```python
from build123d import *

# Parameters (mm, degrees)
F2_R     = 75
F3_DEPTH = 4
F5_R     = 67.5
F6_DEPTH = 12
F8_R     = 75
F9_DEPTH = 4


with BuildPart() as f3:
    # F2 (on Top) → F3 (new body)
    with BuildSketch(Plane.XY):
        Circle(F2_R)
    extrude(amount=F3_DEPTH)

    # F5 (on offset) → F6 (join)
    with BuildSketch(Plane.XY.offset(4)):
        Circle(F5_R)
    extrude(amount=F6_DEPTH)

    # F8 (on offset) → F9 (join)
    with BuildSketch(Plane.XY.offset(16)):
        Circle(F8_R)
    extrude(amount=F9_DEPTH)


with BuildPart() as f10_1:
    # F10: copy of F3
    add(f3.part.moved(Location((0, 0, 20))))


with BuildPart() as f12_1:
    # F12: copy of F3
    add(f3.part)


solid = f3.part
```
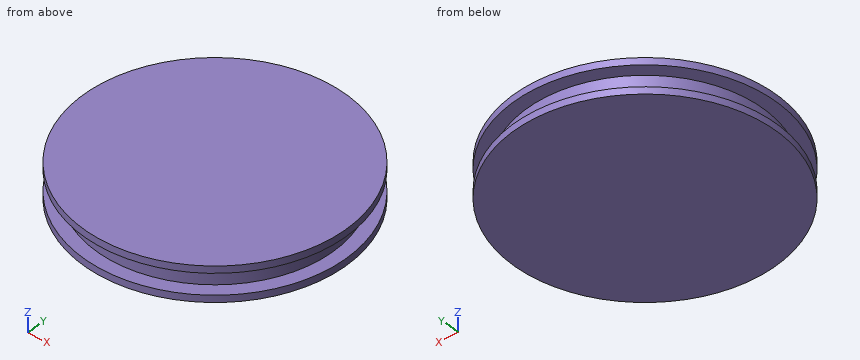
Could you check a few things on this model? Use its own coordinates, in mm. Coordinates: 2 decimals unless noted, no trailing zeros. Loops run counter-clockwise (first coordinate to the right, second up) from the corner with the lowest first, then second, coordinate; pieces in that order, holes last.
1) Please list where these lines run through material, in increasing order: line 1 along Z through (x, y) = (-57.5, 37); line 2 along Y through (x, z) = (-1, 6); line 3 along Y through (x, z) = (14, 8.5).
Reported:
line 1: z = 0 to 4, 16 to 20
line 2: y = -67.49 to 67.49
line 3: y = -66.03 to 66.03
2) Imagine slicing it at C-C (z = 13.5). List the corners of the cut face in (x, y) for me, and give its area (3 significant figures).
Reported:
outline: circle Ø135 at (0, 0)
area: 14,300 mm2
3) Will these pins go through, and if not, where does the flat tip stop? pin 1 Ø2 at (y, z) = (-22.5, 15.5) entering from +X; pin 2 Ø5 at (y, z) = (26.5, 15.5) entering from +X; pin 3 Ø2 at (y, z) = (23, 10) entering from -X.
Reported:
pin 1: stops at x = 71.81
pin 2: stops at x = 71.04
pin 3: stops at x = -63.81
4) Imagine slicing it at A-A (y = 0). List the corners of the cut face in (x, z) for me, and give its area (3 significant figures).
Reported:
outline: (-75, 0) - (75, 0) - (75, 4) - (67.5, 4) - (67.5, 16) - (75, 16) - (75, 20) - (-75, 20) - (-75, 16) - (-67.5, 16) - (-67.5, 4) - (-75, 4) - close
area: 2,820 mm2
